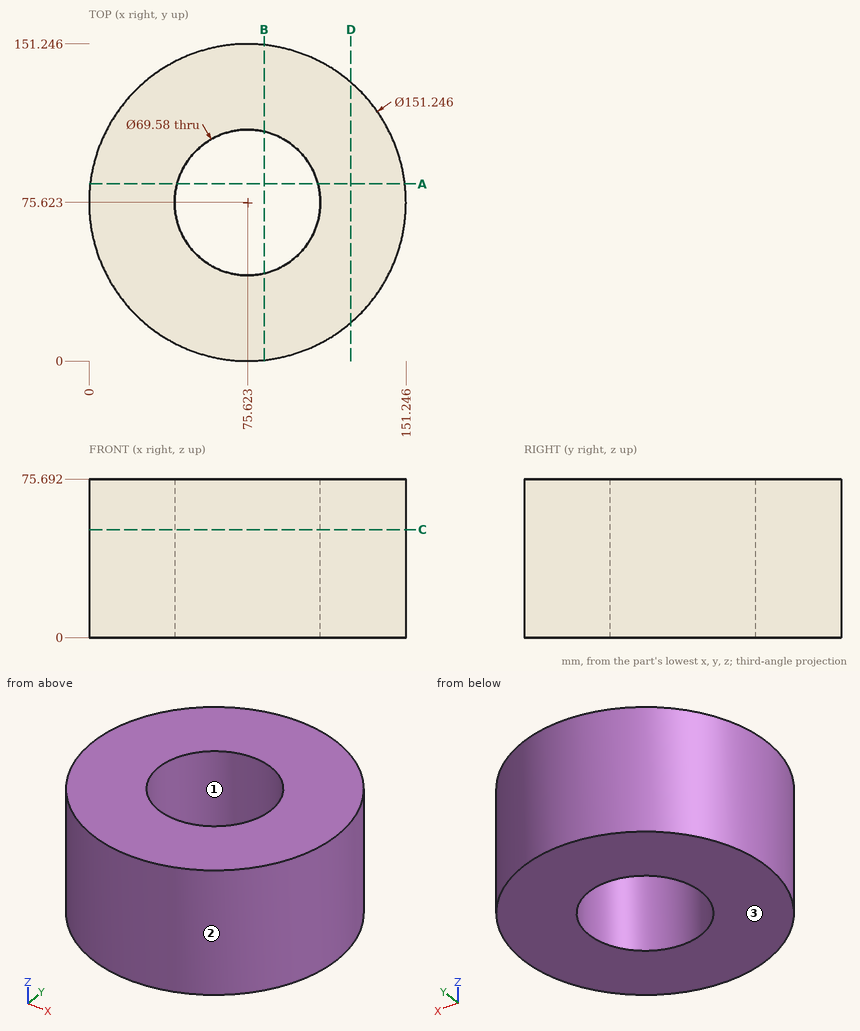
Geometry check sheet. Reference: drawing and pictorial views, mm from the part's lowest x, y, z. Round coordinates to 2 decimals unless told otherwise and drop trailing zeros. Order: outer loops, then holes, each group sorted by start corner. A loop starts at its lowest first (then second) coordinate and runs counter-clockwise, first axis right, second up. Notation, with made-up numbers: M -4,-8 L 1,-8 A28 ccw 1,13 Z; hole C -19.5,20 d4. An arc over 180 degrees is marked long. Answer as CSV lines item,"result".
1) Sectioned sample at B-B on x = 83.5. Record the cut outline in (y, z) (1 decimal), and give its area (3 significant figures).
Entries:
outline,"M 0.4,0 L 41.7,0 L 41.7,75.7 L 0.4,75.7 Z; M 109.5,0 L 150.8,0 L 150.8,75.7 L 109.5,75.7 Z"
area,"6,260 mm2"
2) Sectioned sample at D-D on x = 125. Record the cut outline in (y, z) (1 decimal).
Entries:
outline,"M 18.3,0 L 132.9,0 L 132.9,75.7 L 18.3,75.7 Z"
3) Mould release check, pull along Y, two halves, no side actions. Record for the marked faces 1, 2 and 3: +Y half, -Y half, draft (parallel to the pull), parting line (faces both ways), or undercut.
Entries:
face 1,"undercut"
face 2,"parting line"
face 3,"draft"
4) Gauge pin test, flat ends, axial feed: pin 1 Ø6 at (x, z) = (63.5, 28.5) entering from -Y; pin 2 Ø1 at (x, z) = (39.5, 17.5) entering from -Y (1 decimal); pin 3 Ø1.5 at (x, z) = (46.5, 9) entering from +Y. Record the tip position at first contact, or that the pin passes through.
Entries:
pin 1,"y = 0.55"
pin 2,"y = 8.9"
pin 3,"y = 145.72"
5) Sectioned sample at C-C on z = 51.5. Record the cut outline in (x, y) (1 decimal), and give its area (3 significant figures).
Entries:
outline,"C 75.6,75.6 d151.2; hole C 75.6,75.6 d69.6"
area,"14,200 mm2"
6) Sectioned sample at A-A on y = 84.5. Record the cut outline in (x, z) (1 decimal).
Entries:
outline,"M 0.5,0 L 42,0 L 42,75.7 L 0.5,75.7 Z; M 109.3,0 L 150.7,0 L 150.7,75.7 L 109.3,75.7 Z"
7) Thickness scan on probe 1 along Y at (x, z) = (93, 23.5) (1 decimal); probe 2 along X at (y, z) = (89, 28); probe 3 along X at (y, z) = (51, 16) (1 decimal). Record the ranges inside material, lowest first. Write a range as [from, to].
Entries:
probe 1,"[2, 45.5], [105.8, 149.2]"
probe 2,"[1.19, 43.51], [107.74, 150.05]"
probe 3,"[4.1, 51], [100.2, 147.1]"
